Part model, mm, in its own coordinate system. Coordinates: 2 decimals unless noted, no trailing zeros. Order: outer loops, then holes, each group sorted by start corner. A loop starts at its lowest first (then second) coordinate and runs counter-clockwise, first axis right, second up. Notation, with made-up numbers: (46, -17.5) - (62, -17.5) arc R34 cw to (62, 13.5) - close; hole circle Ø2 at (83.5, 59.5). An arc over 180 degrees is marked (long way). Use a Markdown table: item, result. Add a question column.
1) Saw through at C-C on z = -2.4. Count the separate pieces of the cut face and the enclosed holes in it, then the cut area to 3 significant figures.
2) Wall check: L1, parallel to Y at x = 82.25, z = -0.85; L2, parallel to Y at x = 116.5, z = -2.85; L3, parallel to Y at x = 125, z = -2.4. Give the ranges that are in metal, low to high. Write a range as [from, to].
3) Drop flat-ended pins along their axis: P1, Ø1, axis at y = 65.5, z = -1.5, coming from the +X side; P2, Ø4.5, axis at x = -122.5, y = -20.25, coming from the +Z side. Give the stop position or say it passes through.
4) Saw through at A-A on x = 117.25. List the corners of the cut face in (y, z) (3 decimals), then the cut area to 3 significant figures.
5) Saw through at D-D on y = -59.5. List the corners of the cut face in (x, z) (3 decimals).
6) Saw through at B-B on x = 15. List the corners of the cut face in (y, z) (3 decimals).
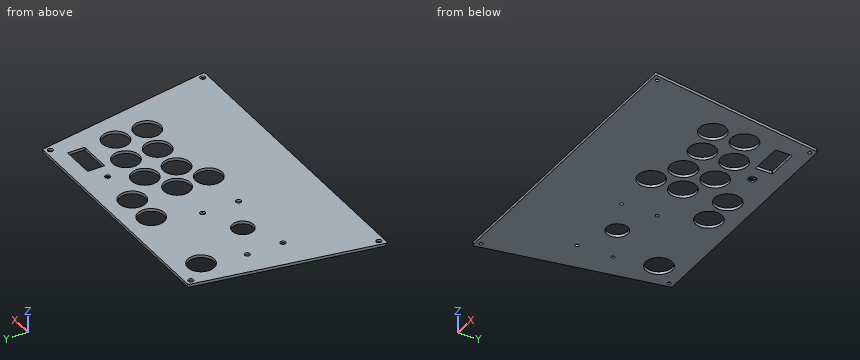
Autodesk Inventor part; units mm, degrees
ref_plane "YZ Plane" through (0, 0, 0) normal (1, 0, 0) x (0, 1, 0)
ref_plane "XZ Plane" through (0, 0, 0) normal (0, 1, 0) x (-1, 0, 0)
ref_plane "XY Plane" through (0, 0, 0) normal (0, 0, 1) x (1, 0, 0)
sketch "Sketch1" plane through (0, 0, 0) normal (0, 0, 1) x (1, 0, 0)
  circle A0 centre (-80, 0) radius 12
  circle A1 centre (15, -18) radius 15
  circle A2 centre (15, 18) radius 15
  circle A3 centre (46.25, 0) radius 15
  circle A4 centre (46.25, 36) radius 15
  circle A5 centre (82.25, 0) radius 15
  circle A6 centre (82.25, 36) radius 15
  circle A7 centre (117.25, -9) radius 15
  circle A8 centre (117.25, 27) radius 15
  line L0 (-175, -108) -> (175, -108)
  line L1 (-175, -108) -> (-138.853, 97)
  line L2 (175, -108) -> (138.853, 97)
  line L3 (-138.853, 97) -> (138.853, 97)
  line L4 (46.25, 36) -> (82.25, 36) construction
  line L5 (82.25, 36) -> (82.25, 0) construction
  line L6 (46.25, 36) -> (46.25, 0) construction
  line L7 (46.25, 0) -> (82.25, 0) construction
  line L8 (117.25, 27) -> (117.25, -9) construction
  line L9 (15, 18) -> (15, -18) construction
  circle A9 centre (18, 67) radius 15
  circle A10 centre (-18, 67) radius 15
  circle A11 centre (-113, 67) radius 15
  line L10 (83, 79) -> (121, 79)
  line L11 (121, 79) -> (121, 59.7)
  line L12 (121, 59.7) -> (83, 59.7)
  line L13 (83, 59.7) -> (83, 79)
  line L14 (0, 97) -> (0, -108) construction
  point P0 (0, 0)
  point P1 (-167.8495, -102)
  point P2 (-133.8184, 91)
  point P3 (167.8495, -102)
  point P4 (133.8184, 91)
  point P5 (-122.5, -20.25)
  point P6 (-37.5, -20.25)
  point P7 (-122.5, 20.25)
  point P8 (-37.5, 20.25)
  dimension "d3" = 24
  dimension "d18" = 30
  dimension "d37" = 90
  dimension "d38" = 80
  dimension "d40" = 80
  dimension "d42" = 350
  dimension "d45" = 31.25
  dimension "d46" = 36
  dimension "d47" = 35
  dimension "d48" = 18
  dimension "d49" = 18
  dimension "d50" = 18
  dimension "d51" = 9
  dimension "d52" = 27
  dimension "d53" = 95
  dimension "d57" = 205
  dimension "d58" = 160
  dimension "d65" = 19.3
  dimension "d66" = 38
  dimension "d67" = 30
  dimension "d73" = 30
  dimension "d74" = 36
  dimension "d76" = 18
  dimension "d77" = 95
  dimension "d78" = 18
  dimension "d79" = 65
  dimension "d92" = 6
  dimension "d93" = 6
  dimension "d94" = 6
  dimension "d95" = 6
  dimension "d96" = 20.25
  dimension "d102" = 42.5
  dimension "d103" = 85
  dimension "d104" = 40.5
extrude "Extrusion5" add sketch "Sketch1" against normal blind 3.175
hole "Hole1" at (-167.8495, -102, 0) at (-133.8184, 91, 0) at (133.8184, 91, 0) at (167.8495, -102, 0) at (-122.5, -20.25, 0) at (-37.5, -20.25, 0) at (-122.5, 20.25, 0) at (-37.5, 20.25, 0) direction (0, 0, -1) diameter 4 end through all countersink diameter 6 countersink angle 90
fillet "Fillet9" radius 2 1 edges at (-138.853, 97, -1.5875)
fillet "Fillet10" radius 2 1 edges at (-175, -108, -1.5875)
fillet "Fillet11" radius 2 1 edges at (175, -108, -1.5875)
fillet "Fillet12" radius 2 1 edges at (138.853, 97, -1.5875)
fillet "Fillet13" radius 0.5 1 edges at (83, 79, -1.5875)
fillet "Fillet14" radius 0.5 1 edges at (121, 79, -1.5875)
fillet "Fillet15" radius 0.5 1 edges at (121, 59.7, -1.5875)
fillet "Fillet16" radius 0.5 1 edges at (83, 59.7, -1.5875)
sketch "Sketch2" plane through (0, 0, -3.175) normal (0, 0, -1) x (-1, 0, 0)
  line L0 (-83, 78.5) -> (-83, 60.2)
  circle A0 centre (-18, 67) radius 15
  point P0 (0, 0)
  point P1 (-65, 67)
  dimension "d130" = 18
hole "Hole3" at (65, 67, -3.175) direction (0, 0, 1) diameter 5.9 end through all counterbore diameter 9 counterbore depth 1.5875
properties part number "Panel_top" material "Aluminum 1100-H18"
Results are:
| question | item | result |
|---|---|---|
| 1 | separate pieces | 1 |
| 1 | enclosed holes | 22 |
| 1 | area | 55,200 mm2 |
| 2 | L1 | [-108, -15], [15, 21], [51, 97] |
| 2 | L2 | [-108, -23.98], [5.98, 12.02], [41.98, 59.7], [79, 97] |
| 2 | L3 | [-108, -21.84], [3.84, 14.16], [39.84, 97] |
| 3 | P1 | x = 144.5 |
| 3 | P2 | z = -0.75 |
| 4 | outline | (-108, -3.175) - (-24, -3.175) - (-24, 0) - (-108, 0) - close; (6, -3.175) - (12, -3.175) - (12, 0) - (6, 0) - close; (42, -3.175) - (59.7, -3.175) - (59.7, 0) - (42, 0) - close; (79, -3.175) - (97, -3.175) - (97, 0) - (79, 0) - close |
| 4 | area | 399 mm2 |
| 5 | outline | (-166.448, -3.175) - (166.448, -3.175) - (166.448, 0) - (-166.448, 0) - close |
| 6 | outline | (-108, -3.175) - (-33, -3.175) - (-33, 0) - (-108, 0) - close; (-3, -3.175) - (3, -3.175) - (3, 0) - (-3, 0) - close; (33, -3.175) - (52.303, -3.175) - (52.303, 0) - (33, 0) - close; (81.697, -3.175) - (97, -3.175) - (97, 0) - (81.697, 0) - close |
